Here's the drawing with two shaded views (mm, measured from the low corner). I have some questions. A direction names the side the tool comes from. Give positions to 0.01 mm unless a question says otherwise; leave off trailing zeros. Write each loop counter-clockwise with the first axis right and the second up, starting at its lowest first coordinate (ties: lowest second). Pieces come first, ordered by that corner, then holes. Notation, with made-up numbers: (59.5, -18.75) - (77.5, -18.75) arc R21 cw to (77.5, -5.75) - close; hole circle Ø3 at (-32.75, 85.5). An arc over 180 degrees is marked (long way). Answer as a JSON object with one key per item and string values. Group by question number.
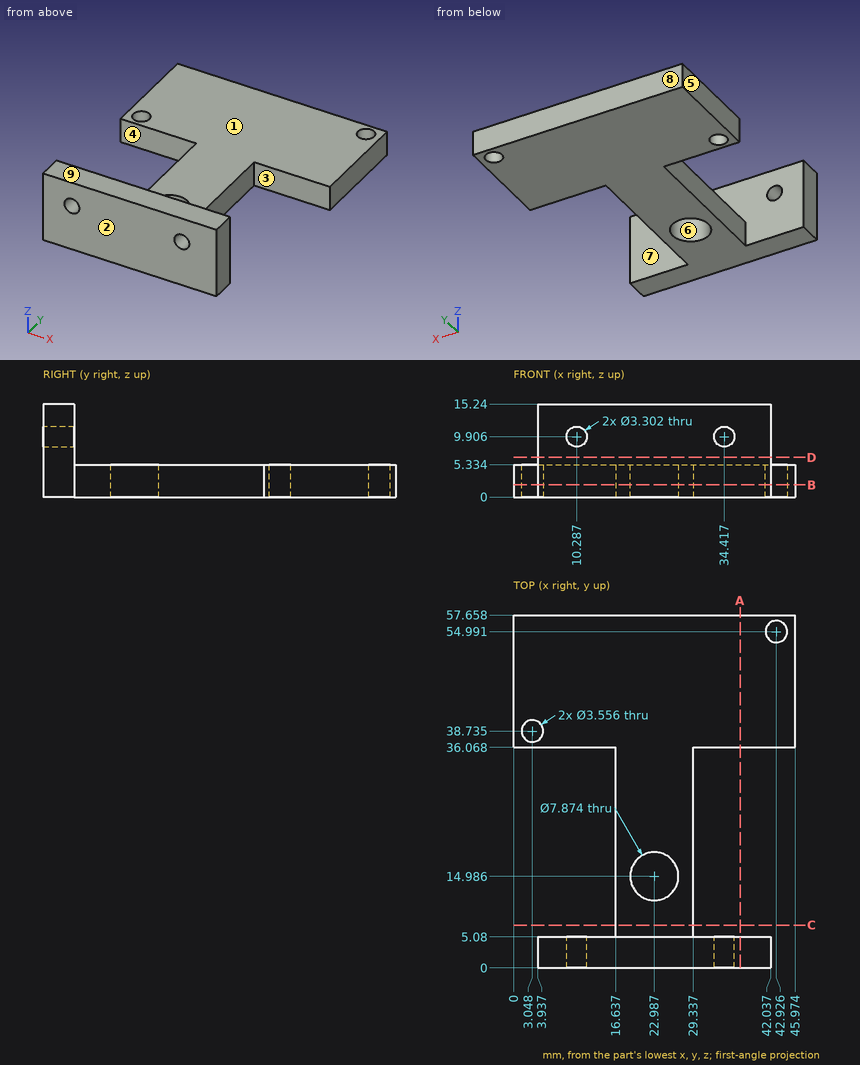
(1) I need wall thicknesses on L1, parallel to Y at x = 16, z = 1.25; L2, parallel to Y at x = 35.5, z = 8.5; L3, parallel to Z at x = 7, y = 49. Which ranges of each line are inside material? Lowest first, please.
(2) I want a section at B-B, the plane z = 2. Please give me the cut outline in (x, y) (3 decimals).
(3) I want a section at A-A, the plane x = 37. Please give me the cut outline in (y, z).
(4) I want a section at D-D, the plane z = 6.5. Please give me the cut outline in (x, y), and give its area (3 significant figures).
(5) I want a section at C-C, the plane y = 7. Please give me the cut outline in (x, z).
(6) For the marked faces 1, 2, 3, 4 and 5, which set-ups out of +Z, -Z, +X, -X, +Y, -Y let a thin tool reach every point of the face, with its end or its side?
(7) If we mould it in two halves opening along Y, with no side actions, what happens to the marked faces 6, 7, 8 and 9? For each: +Y half, -Y half, draft (parallel to the pull), parting line (faces both ways), or undercut.
(8) Will these pins go through, and if not, where does the flat tip stop? P1, Ø3, axis at y = 42.5, z = 7.5, coming from the -X side; P2, Ø7.5, axis at x = 20.5, z = 7.5, coming from the +Y side; P3, Ø4.5, axis at y = 23, z = 2, coming from the -X side; P4, Ø4.5, axis at y = 28, z = 4, coming from the +X side.
Entries:
{
 "1": {"L1": "0 to 5.08, 36.07 to 57.66", "L2": "0 to 5.08", "L3": "0 to 5.33"},
 "2": {"outline": "(0, 36.068) - (16.637, 36.068) - (16.637, 5.08) - (3.937, 5.08) - (3.937, 0) - (42.037, 0) - (42.037, 5.08) - (29.337, 5.08) - (29.337, 36.068) - (45.974, 36.068) - (45.974, 57.658) - (0, 57.658) - close; hole circle Ø3.556 at (3.048, 38.735); hole circle Ø7.874 at (22.987, 14.986); hole circle Ø3.556 at (42.926, 54.991)"},
 "3": {"outline": "(0, 0) - (5.08, 0) - (5.08, 15.24) - (0, 15.24) - close; (36.07, 0) - (57.66, 0) - (57.66, 5.33) - (36.07, 5.33) - close"},
 "4": {"outline": "(3.94, 0) - (42.04, 0) - (42.04, 5.08) - (3.94, 5.08) - close", "area": "194 mm^2"},
 "5": {"outline": "(16.64, 0) - (29.34, 0) - (29.34, 5.33) - (16.64, 5.33) - close"},
 "6": {"face 1": "+Z, +X, -X, +Y", "face 2": "+Z, -Z, +X, -X, -Y", "face 3": "+Z, -Z, +X", "face 4": "+Z, -Z, -X", "face 5": "+Z, -Z, -X, +Y, -Y"},
 "7": {"face 6": "undercut", "face 7": "undercut", "face 8": "+Y half", "face 9": "draft"},
 "8": {"P1": "through", "P2": "y = 57.66", "P3": "x = 16.64", "P4": "x = 29.34"}
}
